The listing builds one solid part. Answer for the finished solid, in the listing's coordinates (mm). Face numbers are marked on the shaded views. A direction names the side the tool comes from. Coordinates: 2 decimals unless noted, no trailing zeros. Loops run counter-clockwise (first coordinate to the right, second up) from the corner with the lowest first, then second, coordinate; pieces in that order, holes last. Notation, with made-up numbers: M 51,81.5 L 92,81.5 A18 ccw 92,85.5 Z; hole C 74,-26.5 d8. An arc over 180 degrees is marked long. Answer as CSV lines item,"result". Start each with the question number.
```python
from build123d import *

# Parameters (mm, degrees)
SKETCH1_R           = 1.27
BOSS_EXTRUDE2_DEPTH = 1.5875
SKETCH2_W           = 15.24
SKETCH2_H           = 1.5875
BOSS_EXTRUDE3_DEPTH = 48.26
SKETCH3_R           = 4.191
CUT_EXTRUDE1_DEPTH  = 2.54
SKETCH4_R           = 1
CUT_EXTRUDE2_DEPTH  = 2.54
SKETCH5_R           = 1
CUT_EXTRUDE3_DEPTH  = 2.54
SKETCH6_R           = 1
CUT_EXTRUDE4_DEPTH  = 2.54


with BuildPart() as part:
    # Sketch1 → Boss-Extrude2 (new body)
    with BuildSketch(Plane(origin=(0, 0, 0), x_dir=(1, 0, 0), z_dir=(0, 1, 0))):
        Polygon((50.8, 0), (50.8, 11.43), (43.18, 24.628227154), (7.62, 24.628227154), (0, 11.43), (0, 0), (17.78, 0), (17.78, -19.327878735), (33.02, -19.327878735), (33.02, 0), align=None)
        with Locations(Location((14.401477372, 11.914121265, 0), (0, 0, 270))):
            Circle(SKETCH1_R, mode=Mode.SUBTRACT)
        with Locations(Location((36.398522628, 11.914121265, 0), (0, 0, 270))):
            Circle(SKETCH1_R, mode=Mode.SUBTRACT)
        with Locations(Location((25.4, -7.135878735, 0), (0, 0, 270))):
            Circle(SKETCH1_R, mode=Mode.SUBTRACT)
    extrude(amount=BOSS_EXTRUDE2_DEPTH)

    # Sketch2 → Boss-Extrude3 (add)
    with BuildSketch(Plane(origin=(0, 1.5875, 0), x_dir=(1, 0, 0), z_dir=(0, 1, 0))):
        with Locations((25.4, -18.534128735)):
            Rectangle(SKETCH2_W, SKETCH2_H)
        Polygon((0, 11.43), (7.62, 24.628227154), (8.994815329, 23.834477154), (1.374815329, 10.63625), align=None)
        Polygon((50.8, 11.43), (43.18, 24.628227154), (41.806418442, 23.835189471), (49.460038325, 10.578730971), align=None)
    extrude(amount=BOSS_EXTRUDE3_DEPTH)

    # Sketch3 → Cut-Extrude1 (cut)
    with BuildSketch(Plane(origin=(0, 1.5875, 0), x_dir=(1, 0, 0), z_dir=(0, 1, 0))):
        with Locations(Location((28.778522628, 17.627987154, 0), (0, 0, 270))):
            Circle(SKETCH3_R)
    extrude(amount=-CUT_EXTRUDE1_DEPTH, mode=Mode.SUBTRACT)

    # Sketch4 → Cut-Extrude2 (cut)
    with BuildSketch(Plane(origin=(43.049335183, 0, -24.854545256), x_dir=(-0.5000000000000016, 0, -0.8660254037844378), z_dir=(0.8660254037844378, 0, -0.5000000000000016))):
        with Locations((-7.881329635, 42.1025)):
            Circle(SKETCH4_R)
        with Locations((-7.881329635, 29.4025)):
            Circle(SKETCH4_R)
    extrude(amount=-CUT_EXTRUDE2_DEPTH, mode=Mode.SUBTRACT)

    # Sketch5 → Cut-Extrude3 (cut)
    with BuildSketch(Plane(origin=(-4.949335183, 0, -2.8575), x_dir=(-0.5000000000000012, 0, 0.866025403784438), z_dir=(-0.8660254037844379, 0, -0.5000000000000011))):
        with Locations((-17.518670365, 42.1025)):
            Circle(SKETCH5_R)
        with Locations((-17.518670365, 29.4025)):
            Circle(SKETCH5_R)
    extrude(amount=-CUT_EXTRUDE3_DEPTH, mode=Mode.SUBTRACT)

    # Sketch6 → Cut-Extrude4 (cut)
    with BuildSketch(Plane.XY.offset(19.327878735)):
        with Locations((25.4, 42.1025)):
            Circle(SKETCH6_R)
        with Locations((25.818223449, 29.4025)):
            Circle(SKETCH6_R)
    extrude(amount=-CUT_EXTRUDE4_DEPTH, mode=Mode.SUBTRACT)


solid = part.part
```
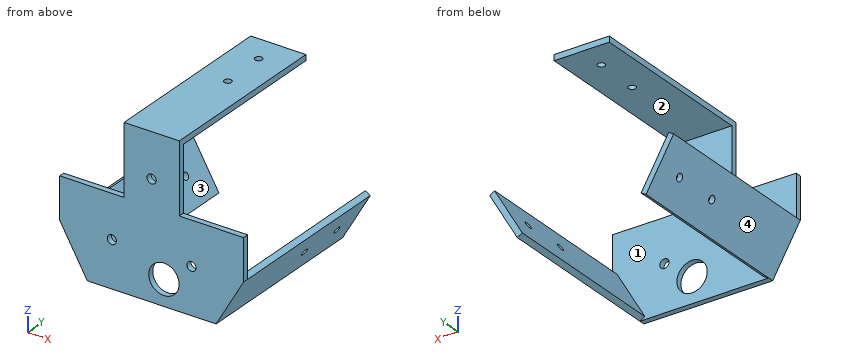
Item 1: For the marked faces 1, 2, 3 and 4, determine the directions among +Z, -Z, +X, -X, +Y, -Y from which every point of the face is accessible in a straight line to the end or side of a thin tool.
Item 2: Section D-D on x = 10 is taken. Determine the outline of the cut face in (y, z).
Item 3: Section B-B on x = 30 is taken. Determine the outline of the cut face in (y, z).
Item 4: Each of these flat-tipped pins is pushed along its axis until it touches: P1, Ø12, axis at x = 7.5, y = 42.5, coming from the +Z side; P2, Ø0.5, axis at x = 9.5, y = 0.5, coming from the +Z side; P3, Ø7.5, axis at x = 22, y = 14, coming from the -Z side; P4, Ø1.8, axis at x = 25.4, y = 42.1, coming from the -Z side. Where does it stop, or does it pass through?
Item 5: Consider line 1 (Z direction, x = 28, y = 31); line 2 (Y direction, x = 31.5, z = 13.5); line 3 (X direction, y = 44, z = -14). Determine where each line is inside the solid, lowest interval first.
Item 6: Section A-A on y = 22.5 is taken. Determine the outline of the cut face in (x, z), then the cut area to 3 significant figures.
Item 7: Section C-C on z = -5 is taken. Determine the outline of the cut face in (x, y).
Results are:
1,face 1,"+Y"
1,face 2,"-Z, +X, -X, +Y"
1,face 3,"+Z, +Y"
1,face 4,"-Z, -X, +Y, -Y"
2,outline,"M 0,-24.63 L 1.59,-24.63 L 1.59,0 L 0,0 Z"
3,outline,"M 0,-24.63 L 1.59,-24.63 L 1.59,-21.64 L 0,-21.64 Z; M 0,-13.62 L 1.59,-13.62 L 1.59,17.74 L 49.85,17.74 L 49.85,19.33 L 0,19.33 Z"
4,P1,"z = -10.85"
4,P2,"z = 0"
4,P3,"z = 17.74"
4,P4,"through"
5,line 1,"17.74 to 19.33"
5,line 2,"0 to 1.59"
5,line 3,"1.48 to 3.32, 47.48 to 49.32"
6,outline,"M 0,-11.43 L 7.62,-24.63 L 8.99,-23.83 L 1.37,-10.64 Z; M 17.78,17.74 L 33.02,17.74 L 33.02,19.33 L 17.78,19.33 Z; M 41.81,-23.84 L 43.18,-24.63 L 50.8,-11.43 L 49.46,-10.58 Z"
6,area,"72.6 mm²"
7,outline,"M 0,0 L 50.8,0 L 50.8,1.59 L 0,1.59 Z"
